Check sheet for the drawn part. Datum: minimum x, y, z corner. Units: mm. Coordinates: 2 decimals unless noted, no trailing zeros. Order: outer loops, then holes, each group sorted by start corner. A loop starts at its lowest first (then second) coordinate and runs counter-clockwise, first axis right, second up.
1. Cross-section at C-C (z = 4.2). Count the separate pieces of the cut face and the enclosed holes in it, then the cut area to 3 significant figures.
2. Cross-section at D-D (y = 17.5). Enter the section's corners in (x, z).
3. Gauge pin test, flat ends, axial feed: pin 1 Ø8.5 at (x, y) = (117.5, 17.5) entering from +Z; pin 2 Ø2 at (x, z) = (58.5, 1.5) entering from +Y. Record the tip position at first contact, or that the pin passes through.
4. Cross-section at B-B (x = 155.5). Enter the section's corners in (y, z).
5. Cross-section at A-A (y = 117.5). Enter the section's corners in (x, z), then the cut area to 3 significant figures.
6. Thickness scan on line 1 (Y direction, x = 117.5, z = 2.9); line 2 (Y direction, x = 116, z = 3.85); line 3 (X direction, y = 158, z = 3.3). Record the ranges inside material, lowest first.
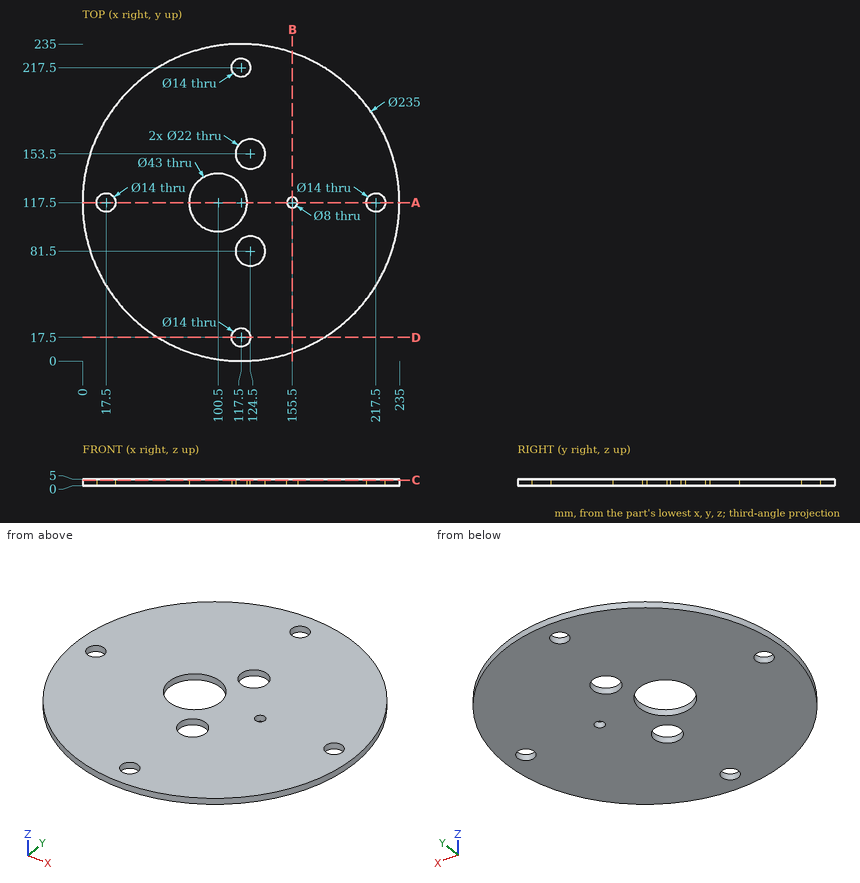
Data:
1. separate pieces: 1
1. enclosed holes: 8
1. area: 40,500 mm2
2. outline: (55.81, 0) - (110.5, 0) - (110.5, 5) - (55.81, 5) - close; (124.5, 0) - (179.19, 0) - (179.19, 5) - (124.5, 5) - close
3. pin 1: passes through
3. pin 2: stops at y = 219.69
4. outline: (6.31, 0) - (113.5, 0) - (113.5, 5) - (6.31, 5) - close; (121.5, 0) - (228.69, 0) - (228.69, 5) - (121.5, 5) - close
5. outline: (0, 0) - (10.5, 0) - (10.5, 5) - (0, 5) - close; (24.5, 0) - (79, 0) - (79, 5) - (24.5, 5) - close; (122, 0) - (151.5, 0) - (151.5, 5) - (122, 5) - close; (159.5, 0) - (210.5, 0) - (210.5, 5) - (159.5, 5) - close; (224.5, 0) - (235, 0) - (235, 5) - (224.5, 5) - close
5. area: 780 mm2
6. line 1: y = 0 to 10.5, 24.5 to 73.01, 89.99 to 104.34, 130.66 to 145.01, 161.99 to 210.5, 224.5 to 235
6. line 2: y = 0.01 to 10.66, 24.34 to 74.52, 88.48 to 102.6, 132.4 to 146.52, 160.48 to 210.66, 224.34 to 234.99
6. line 3: x = 7.2 to 114.46, 134.54 to 227.8
